Geometry check sheet. Reference: the model listing, model coordinates, mm. A direction names the side the tool comes from. Give positions to 0.01 mm unless a question says otherwise; leave off trailing zeros. Write each loop counter-clockwise with the first axis right and the second up, starting at its lowest first coordinate (ties: lowest second). Pieces come first, ordered by that corner, then holes. Notation, with made-up numbers: (18.5, 52.5) - (62.5, 52.5) arc R6 ccw to (62.5, 60.5) - close; hole circle Ø9 at (-24, -21.75). An arc over 180 degrees is marked (long way). Write item = value, one per line. Start each with the question number.
(1) Draft check along X on faces 1 (the flat face through (-29, -42.5, 6)), 2 (the flat face through (-30, 35, 0)), 3 (the flat face through (-36.578, 25.843, 6.439)). Enter one of: pulls with the +X half, pulls with the -X half, needs draft (parallel to the pull), parting line crosses it, or undercut.
(2) Section check B-B, the plane z = 1. Give the number of separate pieces and of enclosed holes in the cut face, plus the area to 3 significant figures.
(3) Thickness scan on L1, parallel to X at y = -31.75, z = 2.75; L2, parallel to Y at x = 29.21, z = 3; L3, parallel to X at y = -5, z = 5.5. Record the ranges inside material, lowest first.
(4) Section check C-C, the plane y = -17.5. Enter the section's corners in (x, z) (3 decimals), plus the area to 3 significant figures.
(5) Section check A-A, the plane x = -4. Enter the section's corners in (y, z) (3 decimals).
(6) Access from +Z, -Z, +X, -X, +Y, -Y to the whole of each face (thin tool, end or side, straight path). Record for faces 4 (the flat face through (30, 23.65, -8)), 5 (the flat face through (-26.5, 0, 8)), 6 (the flat face through (28, 35, 0)).
(7) Section check D-D, the plane y = -31.75. Enter the section's corners in (x, z).
(8) Depth check by flat-ended pin: pin 1 Ø7.5 at (x, z) = (-30.5, -8.5) entering from +Y; pin 2 Ø5.5 at (x, z) = (-29.5, -11.5) entering from -Y; pin 3 Ø12 at (x, z) = (-5.5, -11.5) entering from -Y. Enter the tip coordinate at first touch or a pass-through.
```python
from build123d import *

# Parameters (mm, degrees)
F0_W      = 80
F0_H      = 85
F1_DEPTH  = 25.4
F2_W      = 53
F2_H      = 17
F3_DEPTH  = 27.7749
F4_W      = 80
F4_H      = 85
F5_DEPTH  = 12.7
F6_R      = 3.1623
F7_DEPTH  = 22.86
F8_W      = 25.4
F8_H      = 5.08
F9_DEPTH  = 25.4
F10_R     = 7.62
F11_R     = 7.62
F12_R     = 7.62
F13_R     = 7.62
F15_DEPTH = 16.51
F16_W     = 35
F16_H     = 50.8
F17_DEPTH = 25.4
F19_DEPTH = 38.1
F20_R     = 6.35
F20_R_2   = 3.81
F21_DEPTH = 6.35
F23_DEPTH = 29.21
F25_DEPTH = 25.4


with BuildPart() as f1:
    # F0 (on Top) → F1 (new body)
    with BuildSketch(Plane.XY):
        Rectangle(F0_W, F0_H)
    extrude(amount=F1_DEPTH)

    # F2 (on Front) → F3 (cut, symmetric)
    with BuildSketch(Plane.XZ):
        with Locations((0, 12.065)):
            Rectangle(F2_W, F2_H)
    extrude(amount=F3_DEPTH, both=True, mode=Mode.SUBTRACT)

    # F4 (on face) → F5 (cut)
    with BuildSketch(Plane.XY.offset(25.4)):
        Rectangle(F4_W, F4_H)
    extrude(amount=-F5_DEPTH, mode=Mode.SUBTRACT)

    # F6 (on face) → F7 (join)
    with BuildSketch(Plane(origin=(0, 0, 0), x_dir=(1, 0, 0), z_dir=(0, 0, -1))):
        with Locations((-29.21, 31.75)):
            Circle(F6_R)
        with Locations((29.21, 31.75)):
            Circle(F6_R)
        with Locations((29.21, -31.75)):
            Circle(F6_R)
        with Locations((-29.21, -31.75)):
            Circle(F6_R)
    extrude(amount=F7_DEPTH)

    # F8 (on face) → F9 (cut)
    with BuildSketch(Plane.XY.offset(3.565)):
        with Locations((0, -19.05)):
            Rectangle(F8_W, F8_H)
    extrude(amount=-F9_DEPTH, mode=Mode.SUBTRACT)

    # F10
    f10_edges = [f1.edges().sort_by_distance(p)[0] for p in [
        (-40, -42.5, 6.35),
    ]]
    fillet(f10_edges, radius=F10_R)

    # F11
    f11_edges = [f1.edges().sort_by_distance(p)[0] for p in [
        (-40, 42.5, 6.35),
    ]]
    fillet(f11_edges, radius=F11_R)

    # F12
    f12_edges = [f1.edges().sort_by_distance(p)[0] for p in [
        (40, 42.5, 6.35),
    ]]
    fillet(f12_edges, radius=F12_R)

    # F13
    f13_edges = [f1.edges().sort_by_distance(p)[0] for p in [
        (40, -42.5, 6.35),
    ]]
    fillet(f13_edges, radius=F13_R)

    # F14 (on face) → F15 (join)
    with BuildSketch(Plane(origin=(0, 0, 0), x_dir=(1, 0, 0), z_dir=(0, 0, -1))):
        Polygon((-19.2960512242, 16.4658580638), (-26.4802561211, 23.6500629607), (-34.1002561211, 23.6500629607), (-34.1002561211, 18.5700629607), (-26.4802561211, 18.5700629607), (-24.3760512242, 16.4658580638), (-24.3760512242, 8.2329290319), (-24.3760512242, 0), (-24.3760512242, -8.2329290319), (-24.3760512242, -16.4658580638), (-26.4802561211, -18.5700629607), (-34.1002561211, -18.5700629607), (-34.1002561211, -23.6500629607), (-26.4802561211, -23.6500629607), (-19.2960512242, -16.4658580638), (-17.5, -14.6698068396), (-17.5, 0), (-17.5, 14.6698068396), align=None)
        Polygon((19.2960498, -16.4658578227), (26.4802546969, -23.6500627196), (34.1002546969, -23.6500627196), (34.1002546969, -18.5700627196), (26.4802546969, -18.5700627196), (24.3760498, -16.4658578227), (24.3760498, -8.2329287908), (24.3760498, 2.411e-07), (24.3760498, 8.232929273), (24.3760498, 16.4658583049), (26.4802546969, 18.5700632018), (34.1002546969, 18.5700632018), (34.1002546969, 23.6500632018), (26.4802546969, 23.6500632018), (19.2960498, 16.4658583049), (17.5, 14.6698068396), (17.5, 0), (17.5, -14.6698068396), align=None)
    extrude(amount=F15_DEPTH)

    # F16 (on face) → F17 (cut)
    with BuildSketch(Plane(origin=(0, 0, 0), x_dir=(1, 0, 0), z_dir=(0, 0, -1))):
        Rectangle(F16_W, F16_H)
    extrude(amount=F17_DEPTH, mode=Mode.SUBTRACT)

    # F18 (on face) → F19 (cut, symmetric)
    with BuildSketch(Plane.XY.offset(3.565)):
        Polygon((-26.5, -42.5), (26.5, -42.5), (22.69, -35.13745), (-22.69, -35.13745), align=None)
        Polygon((33.3297468424, -24.0099126621), (40, -27.7749), (40, 27.7749), (33.25, 23.9649), align=None)
        Polygon((-26.5, 42.5), (-22.69, 35.13745), (22.69, 35.13745), (26.5, 42.5), align=None)
        Polygon((-33.25, -23.9649), (-33.25, 23.9649), (-40, 27.7749), (-40, -27.7749), align=None)
    extrude(amount=F19_DEPTH, both=True, mode=Mode.SUBTRACT)

    # F20 (on face) → F21 (cut)
    with BuildSketch(Plane(origin=(0, 0, 0), x_dir=(1, 0, 0), z_dir=(0, 0, -1))):
        with Locations((-29.21, 31.75)):
            Circle(F20_R)
        with Locations((-29.21, 31.75)):
            Circle(F20_R_2, mode=Mode.SUBTRACT)
        with Locations((29.21, 31.75)):
            Circle(F20_R)
        with Locations((29.21, 31.75)):
            Circle(F20_R_2, mode=Mode.SUBTRACT)
        with Locations((29.21, -31.75)):
            Circle(F20_R)
        with Locations((29.21, -31.75)):
            Circle(F20_R_2, mode=Mode.SUBTRACT)
        with Locations((-29.21, -31.75)):
            Circle(F20_R)
        with Locations((-29.21, -31.75)):
            Circle(F20_R_2, mode=Mode.SUBTRACT)
    extrude(amount=-F21_DEPTH, mode=Mode.SUBTRACT)

    # F22 (on face) → F23 (join)
    with BuildSketch(Plane.XY.offset(12.7)):
        Polygon((22.69, -35.13745), (-22.69, -35.13745), (-17.7075349979, -42.5), (17.7075349979, -42.5), align=None)
        Polygon((-17.7075349979, 42.5), (-22.69, 35.13745), (22.69, 35.13745), (17.7075349979, 42.5), align=None)
    extrude(amount=-F23_DEPTH)

    # F24 (on face) → F25 (cut)
    with BuildSketch(Plane(origin=(0, 0, -16.51), x_dir=(1, 0, 0), z_dir=(0, 0, -1))):
        Polygon((17.7075349979, 42.5), (-17.7075349979, 42.5), (-8.8537674989, 38.818725), (0, 38.818725), (8.8537674989, 38.818725), align=None)
    extrude(amount=-F25_DEPTH, mode=Mode.SUBTRACT)


solid = f1.part
```
Model answer:
q1.face_1 = needs draft
q1.face_2 = undercut
q1.face_3 = pulls with the -X half
q2.separate_pieces = 5
q2.enclosed_holes = 5
q2.area = 5,370 mm²
q3.L1 = -40 to -35.56, -33.02 to -25.4, -22.86 to 22.86, 25.4 to 33.02, 35.56 to 40
q3.L2 = -42.5 to -38.1, -35.56 to -27.94, -25.4 to 25.4, 27.94 to 35.56, 38.1 to 42.5
q3.L3 = -33.25 to -26.5, 26.5 to 33.3
q4.outline = (-33.25, 0) - (-25.41, 0) - (-25.41, -16.51) - (-20.33, -16.51) - (-20.33, 0) - (-12.7, 0) - (-12.7, 3.565) - (-26.5, 3.565) - (-26.5, 12.7) - (-33.25, 12.7) - close; (12.7, 0) - (20.33, 0) - (20.33, -16.51) - (25.41, -16.51) - (25.41, 0) - (33.319, 0) - (33.319, 12.7) - (26.5, 12.7) - (26.5, 3.565) - (12.7, 3.565) - close
q4.area = 438 mm²
q5.outline = (-42.5, 8.89) - (-38.819, 8.89) - (-38.819, -16.51) - (-35.137, -16.51) - (-35.137, 0) - (-21.59, 0) - (-21.59, 3.565) - (-27.775, 3.565) - (-27.775, 12.7) - (-42.5, 12.7) - close; (-16.51, 0) - (35.137, 0) - (35.137, -16.51) - (42.5, -16.51) - (42.5, 12.7) - (27.775, 12.7) - (27.775, 3.565) - (-16.51, 3.565) - close
q6.face_4 = -Z, +X, -X
q6.face_5 = +Z
q6.face_6 = -Z
q7.outline = (-40, 0) - (-35.56, 0) - (-35.56, 6.35) - (-33.02, 6.35) - (-33.02, 0) - (-32.37, 0) - (-32.37, -22.86) - (-26.05, -22.86) - (-26.05, 0) - (-25.4, 0) - (-25.4, 6.35) - (-22.86, 6.35) - (-22.86, 0) - (22.86, 0) - (22.86, 6.35) - (25.4, 6.35) - (25.4, 0) - (26.05, 0) - (26.05, -22.86) - (32.37, -22.86) - (32.37, 0) - (33.02, 0) - (33.02, 6.35) - (35.56, 6.35) - (35.56, 0) - (40, 0) - (40, 12.7) - (-40, 12.7) - close
q8.pin_1 = 34.91
q8.pin_2 = -34.91
q8.pin_3 = -39.92
